Read the model definition and answer for the solid it produces. Units are mm, in the model's axes. A direction names the side the tool comes from. Give positions to 0.01 mm unless a question says otherwise; leave off trailing zeros. Loops run counter-clockwise (first coordinate to the right, second up) from the corner with the lowest first, then second, coordinate; pieces in that order, holes last. Notation, with made-up numbers: (28.25, 36.5) -> (79.25, 36.5) arc R27 ccw to (79.25, 65.5) -> close; hole circle Ø4 at (-4.5, 86). An arc over 180 degrees is marked (long way). Answer as CSV lines item,"result". Start each with the question number.
Autodesk Inventor part; units mm, degrees
ref_plane "YZ Plane" through (0, 0, 0) normal (1, 0, 0) x (0, 1, 0)
ref_plane "XZ Plane" through (0, 0, 0) normal (0, 1, 0) x (-1, 0, 0)
ref_plane "XY Plane" through (0, 0, 0) normal (0, 0, 1) x (1, 0, 0)
sketch "Sketch1" plane through (0, 0, 0) normal (0, 0, 1) x (1, 0, 0)
  line L0 (-25.1968, 0) -> (-25.1968, -2.9718)
  line L1 (-25.1968, -2.9718) -> (-14.7402, -2.9718)
  line L2 (25.1968, 0) -> (25.1968, -2.9718)
  line L3 (25.1968, -2.9718) -> (14.7402, -2.9718)
  line L4 (-25.1968, 0) -> (-15.0368, 0)
  line L5 (15.0368, 0) -> (25.1968, 0)
  circle A0 centre (0, 0) radius 12.4968
  arc A1 (15.0368, 0) -> (-15.0368, 0) centre (0, 0) ccw
  arc A2 (-14.7402, -2.9718) -> (14.7402, -2.9718) centre (0, 0) ccw
  point P0 (-12.4968, 0)
  dimension "d12" = 24.9936
  dimension "d4" = 2.9718
  dimension "d5" = 2.9718
  dimension "d6" = 50.3936
  dimension "d9" = 12.7
  dimension "d13" = 15.0368
  dimension "d14" = 15.0368
  dimension "d15" = 10.4566
  dimension "d16" = 10.4566
  dimension "d17" = 10.16
extrude "Extrusion2" add sketch "Sketch1" along normal blind 53.975
sketch "Sketch2" plane through (0, 0, 53.975) normal (0, 0, 1) x (1, 0, 0)
  circle A0 centre (0, 0) radius 3.556
  circle A1 centre (0, 0) radius 15.0368
  dimension "d20" = 7.112
  dimension "d21" = 30.0736
extrude "Extrusion3" add sketch "Sketch2" along normal blind 1.905
sketch "Sketch3" plane through (0, 0, 55.88) normal (0, 0, 1) x (1, 0, 0)
  circle A0 centre (0, 0) radius 12.4968
  circle A1 centre (-8.4968, 0) radius 1.25
  circle A2 centre (8.4968, 0) radius 1.25
  dimension "d25" = 2.5
  dimension "d26" = 8.4968
  dimension "d27" = 2.5
  dimension "d28" = 8.4968
extrude "Extrusion4" cut sketch "Sketch3" against normal blind 254 contours A1 | A2
properties part number "Attachment2"
(1) The mould has two halves that part along Y. Classify faces 4 (the face through (-8, -10, 0)), 5 (the face through (-0.77, 3.47, 54.91)), 6 (the face through (-20, 0, 27)): pulls with the +Y half, pulls with the -Y half, needs draft (parallel to the pull), parting line crosses it, or undercut.
(2) A tool of negligible diameter and unlimited length cuts with its end or side. For faces 1 (the face through (11.92, -3.75, 26.61)), 2 (the face through (-20, -2.972, 27)), 3 (the face through (20, 0, 27)), from which of +Z, -Z, +X, -X, +Y, -Y can it reach the whole face along a straight path? Write none if from no direction.
(3) Find section A-A on x = 0. Write down the section's boundary in (y, z) (3 decimals), then the cut area to 3 significant figures.
(4) Each of these flat-tipped pins is pushed along its axis until it touches: P1, Ø1.5, axis at y = -3, z = 36.5, coming from the +X side; P2, Ø7.5, axis at x = -1, y = 2, coming from the -Z side (3 decimals); P3, Ø2, axis at x = -7, z = 41, coming from the -Y side; P4, Ø5, axis at x = -18.5, z = 27.5, coming from the +Y side. Where does it stop, or does it pass through?
(5) Find section C-C on y = -10. Write down the section's boundary in (x, z) (3 decimals), then the cut area to 3 significant figures.
(6) Find section B-B on z = 38. Write down the section's boundary in (x, y), then the cut area to 3 significant figures.
(7) Find the intervals of material crossed by line 1 along X through (y, z) = (-11.5, 10.5); line 2 along Z through (x, y) = (-6.5, -8) (3 decimals); line 3 along Y through (x, z) = (21, 31), in increasing order. Write a range as from..to.
(8) Find section D-D on y = 8. Write down the section's boundary in (x, z) (3 decimals), then the cut area to 3 significant figures.
Answer block:
1,face 4,"needs draft"
1,face 5,"undercut"
1,face 6,"pulls with the +Y half"
2,face 1,"-Z"
2,face 2,"+Z, -Z, -X, -Y"
2,face 3,"+Z, -Z, +X, +Y"
3,outline,"(-15.037, 0) -> (-12.497, 0) -> (-12.497, 53.975) -> (-3.556, 53.975) -> (-3.556, 55.88) -> (-15.037, 55.88) -> close; (3.556, 53.975) -> (12.497, 53.975) -> (12.497, 0) -> (15.037, 0) -> (15.037, 55.88) -> (3.556, 55.88) -> close"
3,area,"318 mm2"
4,P1,"stops at x = 25.2"
4,P2,"stops at z = 53.975"
4,P3,"stops at y = -13.79"
4,P4,"stops at y = 0"
5,outline,"(-11.23, 0) -> (-7.495, 0) -> (-7.495, 53.975) -> (7.495, 53.975) -> (7.495, 0) -> (11.23, 0) -> (11.23, 55.88) -> (-11.23, 55.88) -> close"
5,area,"446 mm2"
6,outline,"(-25.2, -2.97) -> (-14.74, -2.97) arc R15.04 ccw to (14.74, -2.97) -> (25.2, -2.97) -> (25.2, 0) -> (15.04, 0) arc R15.04 ccw to (-15.04, 0) -> (-25.2, 0) -> close; hole circle Ø24.99 at (0, 0)"
6,area,"281 mm2"
7,line 1,"x = -9.69..-4.89, 4.89..9.69"
7,line 2,"z = 53.975..55.88"
7,line 3,"y = -2.97..0"
8,outline,"(-12.732, 0) -> (-9.601, 0) -> (-9.601, 53.975) -> (9.601, 53.975) -> (9.601, 0) -> (12.732, 0) -> (12.732, 55.88) -> (-12.732, 55.88) -> close"
8,area,"387 mm2"
